Build history of the part. All positions in model axes, mm. A direction names the side the tool comes from. Coordinates: 2 decimals unless noted, no trailing zeros. Loops run counter-clockwise (first coordinate to the right, second up) from the corner with the lowest first, then second, coordinate; pieces in that order, holes last.
Item 1: Mould opens along Z. For faces 1 (the face through (-45.675, -4, 32)), 2 (the face through (-41.572, -3.757, 25.615)), 3 (the face through (-44.37, -3.76, -75.57)), 4 (the face through (-44, -3.8, -67.5)) say: released by +Z, released by -Z, zero draft, split by the parting line, or undercut.
Item 2: Cut at C-C (z = -13). List the corners of the cut face in (x, y), and give its area (3 significant figures).
Item 3: Cut at D-D (z = -29). List the corners of the cut face in (x, y), and give its area (3 significant figures).
Item 4: Drill centre lines: line 1 along Z through (x, y) = (-49.75, -1.75); line 2 along Z through (x, y) = (-41.5, -3); line 3 along X through (y, z) = (-2, -55). Where is each one in solid material? Low to high.
Item 5: Cut at B-B (x = -44). List the corners of the cut face in (y, z), and give its area (3 significant figures).
Item 6: 3-axis set-ups, long thin cutter, end or side, ignore diameter. For faces 5 (the face through (-47.76, -3.76, -73.37)), 6 (the face through (-50.61, -3.76, 28.29)), 7 (the face through (-37.598, -4, 32)): which of +Z, -Z, +X, -X, +Y, -Y reach the whole face in a straight line?
Item 7: Flat gauge pins, fed straight in: pin 1 (1.5 mm diameter, centred on y = -3, z = -26, fed in from -X); pin 2 (4 mm diameter, centred on y = -4, z = 31.5, fed in from +X); pin 3 (2.5 mm diameter, centred on y = -4, z = 33.5, fed in from -X). Where does each tip first touch, or does it go through?
Item 8: Cut at A-A (y = -1.5). List the corners of the cut face in (x, z).
from build123d import *

# Parameters (mm, degrees)
F1_DEPTH = 6.35
F2_DEPTH = 7.62


with BuildPart() as f1:
    # F0 (on Front) → F1 (new body)
    with BuildSketch(Plane.XZ):
        with BuildLine():
            Line((-39.743337, -65.643214), (-39.743337, -65.434216))
            Line((-39.743337, -65.434216), (-37.598322, 20.518023))
            Line((-37.598322, 20.518023), (-45.673008, 20.719534))
            Line((-45.673008, 20.719534), (-47.674275, -65.06083))
            ThreePointArc((-47.674275, -65.06083), (-43.623463, -64.189814), (-39.743337, -65.643214))
        make_face()
    extrude(amount=F1_DEPTH)

    # F0 (on Front) → F2 (join)
    with BuildSketch(Plane.XZ):
        with BuildLine():
            Line((-39.743337, -65.643214), (-39.743337, -65.434216))
            Line((-39.743337, -65.434216), (-37.598322, 20.518023))
            Line((-37.598322, 20.518023), (-45.673008, 20.719534))
            Line((-45.673008, 20.719534), (-47.674275, -65.06083))
            ThreePointArc((-47.674275, -65.06083), (-43.623463, -64.189814), (-39.743337, -65.643214))
        make_face()
        with BuildLine():
            Line((-45.673008, 20.719534), (-37.598322, 20.518023))
            ThreePointArc((-37.598322, 20.518023), (-32.601753, 27.984673), (-37.598322, 35.451324))
            Line((-37.598322, 35.451324), (-37.598322, 27.525249))
            ThreePointArc((-37.598322, 27.525249), (-41.636713, 25.615004), (-45.675104, 27.525249))
            Line((-45.675104, 27.525249), (-45.675104, 35.602449))
            ThreePointArc((-45.675104, 35.602449), (-50.610258, 28.160296), (-45.673008, 20.719534))
        make_face()
        with BuildLine():
            ThreePointArc((-36.79691, -71.536034), (-37.574567, -68.241844), (-39.743337, -65.643214))
            ThreePointArc((-39.743337, -65.643214), (-43.623463, -64.189814), (-47.674275, -65.06083))
            ThreePointArc((-47.674275, -65.06083), (-47.930751, -77.865437), (-36.79691, -71.536034))
        make_face()
        Polygon((-46.248433, -67.364986), (-41.593438, -67.644394), (-39.507915, -71.815443), (-42.077387, -75.707083), (-46.732383, -75.427675), (-48.817906, -71.256626), align=None, mode=Mode.SUBTRACT)
    extrude(amount=F2_DEPTH)


solid = f1.part
Filled sheet:
1. face 1: zero draft
1. face 2: released by +Z
1. face 3: undercut
1. face 4: undercut
2. outline: (-46.46, -7.62) - (-38.43, -7.62) - (-38.43, 0) - (-46.46, 0) - close
2. area: 61.1 mm2
3. outline: (-46.83, -7.62) - (-38.83, -7.62) - (-38.83, 0) - (-46.83, 0) - close
3. area: 61.0 mm2
4. line 1: z = -76.34 to -66.74, 24.53 to 31.79
4. line 2: z = -78.4 to -74.83, -67.83 to 25.62
4. line 3: x = -47.44 to -39.48
5. outline: (-7.62, -78.9) - (0, -78.9) - (0, -75.59) - (-7.62, -75.59) - close; (-7.62, -67.5) - (0, -67.5) - (0, 26.18) - (-7.62, 26.18) - close
5. area: 739 mm2
6. face 5: +Y, -Y
6. face 6: -X, +Y, -Y
6. face 7: +Z, +Y, -Y
7. pin 1: stops at x = -46.78
7. pin 2: stops at x = -32.75
7. pin 3: stops at x = -49.5
8. outline: (-47.67, -65.06) arc R7.37 ccw (long way) to (-36.8, -71.54) arc R7.37 ccw to (-39.74, -65.64) - (-39.74, -65.43) - (-37.6, 20.52) arc R8.08 ccw to (-37.6, 35.45) - (-37.6, 27.53) arc R5.22 cw to (-45.68, 27.53) - (-45.68, 35.6) arc R8.08 ccw to (-45.67, 20.72) - close; hole (-48.82, -71.26) - (-46.73, -75.43) - (-42.08, -75.71) - (-39.51, -71.82) - (-41.59, -67.64) - (-46.25, -67.36) - close
